```python
from build123d import *

# Parameters (mm, degrees)
SKETCH1_W                  = 38.1
SKETCH1_H                  = 127
EXTRUDE1_DEPTH             = 3.175
F_4_CLEARANCE_HOLE1_D      = 3.2639
F_4_CLEARANCE_HOLE1_DEPTH  = 101.6
F_4_CLEARANCE_HOLE1_TIP    = 0.980574487
SKETCH4_W                  = 6.35
SKETCH4_H                  = 19.05
CUT_EXTRUDE1_DEPTH         = 79.60930686
TAP_DRILL_FOR_6_TAP1_D     = 2.7051
TAP_DRILL_FOR_6_TAP1_DEPTH = 3.302
TAP_DRILL_FOR_6_TAP1_TIP   = 0.81269403
FILLET1_R                  = 6.35


with BuildPart() as part:
    # Sketch1 → Extrude1 (new body)
    with BuildSketch(Plane(origin=(0, 0, 0), x_dir=(1, 0, 0), z_dir=(0, 1, 0))):
        with Locations((0, -12.7)):
            Rectangle(SKETCH1_W, SKETCH1_H)
    extrude(amount=EXTRUDE1_DEPTH)

    # #4 Clearance Hole1
    with Locations(Plane(origin=(-10.8585, 0, 28.575), x_dir=(0, 0, -1), z_dir=(0, -1, 0))):
        with Locations((0, 0), (0, 21.717), (-38.1, 0), (-38.1, 21.717)):
            Hole(F_4_CLEARANCE_HOLE1_D / 2, depth=F_4_CLEARANCE_HOLE1_DEPTH)
            with Locations((0, 0, -(F_4_CLEARANCE_HOLE1_DEPTH + F_4_CLEARANCE_HOLE1_TIP / 2))):  # 118° drill point
                Cone(0, F_4_CLEARANCE_HOLE1_D / 2, F_4_CLEARANCE_HOLE1_TIP, mode=Mode.SUBTRACT)

    # Sketch4 → Cut-Extrude1 (cut, through all)
    with BuildSketch(Plane.XZ):
        with Locations((-15.875, -41.275)):
            Rectangle(SKETCH4_W, SKETCH4_H)
        with Locations((15.875, -41.275)):
            Rectangle(SKETCH4_W, SKETCH4_H)
    extrude(amount=-CUT_EXTRUDE1_DEPTH, mode=Mode.SUBTRACT)

    # Tap Drill for #6 Tap1
    with Locations(Plane(origin=(-6.35, 3.175, -38.1), x_dir=(0, 0, 1), z_dir=(0, 1, 0))):
        with Locations((0, 0), (0, 12.7)):
            Hole(TAP_DRILL_FOR_6_TAP1_D / 2, depth=TAP_DRILL_FOR_6_TAP1_DEPTH)
            with Locations((0, 0, -(TAP_DRILL_FOR_6_TAP1_DEPTH + TAP_DRILL_FOR_6_TAP1_TIP / 2))):  # 118° drill point
                Cone(0, TAP_DRILL_FOR_6_TAP1_D / 2, TAP_DRILL_FOR_6_TAP1_TIP, mode=Mode.SUBTRACT)

    # Fillet1
    fillet1_edges = [part.edges().sort_by_distance(p)[0] for p in [
        (-12.7, 1.5875, -31.75),
        (12.7, 1.5875, -31.75),
    ]]
    fillet(fillet1_edges, radius=FILLET1_R - 0.0001)  # a hair under: the kernel refuses the full size


solid = part.part
```
The listing builds one solid part. Answer for the finished solid, in the listing's coordinates (mm). A direction names the side the tool comes from. Give positions to 0.01 mm unless a question says otherwise; leave off trailing zeros. Order: outer loops, then holes, each group sorted by start corner. A loop starts at its lowest first (then second) coordinate and runs counter-clockwise, first axis right, second up. Notation, with made-up numbers: (-23.75, 80) -> (-14.75, 80) arc R26 cw to (-14.75, 115) -> close; hole circle Ø7 at (40, 11). An arc over 180 degrees is marked (long way). Write each question's results on one line, items separated by ' | '.
Q1. The part is cut by section A-A, the plane x = -6.35. Give the vertices of the cut face in (y, z) (3 decimals), and give its area (3 significant figures).
Checked values:
outline: (0, -50.8) -> (3.175, -50.8) -> (3.175, -39.453) -> (0, -39.453) -> close; (0, -36.747) -> (3.175, -36.747) -> (3.175, 76.2) -> (0, 76.2) -> close | area: 395 mm^2
Q2. Straight lines are drawn through the part: probe 1 along Z at (x, y) = (-9.5, 2.65); probe 2 along X at (y, z) = (1.5, -41.5); probe 3 along Z at (x, y) = (12, 2.05). For each, find the intervals that lie inside material, in ascending order. Write a range as from..to.
Checked values:
probe 1: z = -50.8..27.67, 29.48..65.77, 67.58..76.2 | probe 2: x = -12.7..12.7 | probe 3: z = -50.8..27.41, 29.74..65.51, 67.84..76.2
Q3. The part is cut by section B-B, the plane y = 1.9. State how many separate pieces and enclosed holes the cut face has, and give its area (3 significant figures).
Checked values:
separate pieces: 1 | enclosed holes: 6 | area: 4,570 mm^2
Q4. The part is cut by section C-C, the plane x = -14. Give the vertices of the cut face in (y, z) (3 decimals).
Checked values:
outline: (0, -34.25) -> (3.175, -34.25) -> (3.175, 76.2) -> (0, 76.2) -> close
Q5. Which of the six approach directions +Z, -Z, +X, -X, +Y, -Y give full straight-line access (tool end or side, diameter ignored) to faces 5 (the face through (12.7, 2, -45)), 6 (the face through (-12.7, 2, -45)), 7 (the face through (-19.05, 2, 23))?
Checked values:
face 5: -Z, +X, +Y, -Y | face 6: -Z, -X, +Y, -Y | face 7: +Z, -Z, -X, +Y, -Y
Q6. Determine the mould class of faces 1 (the face through (-6.87, 1.57, -39.35)), 2 (the face through (-14.61, 1.61, -33.56)), 3 (the face through (14.61, 1.61, -33.56)), 4 (the face through (0, 0, 12)) for opening direction X: pulls with the +X half, pulls with the -X half, needs draft (parallel to the pull), parting line crosses it, or undercut.
Checked values:
face 1: undercut | face 2: pulls with the -X half | face 3: pulls with the +X half | face 4: needs draft
Q7. Each of these flat-tipped pins is pushed along its axis until it touches: P1, Ø2, axis at x = 6.35, z = -38.1, coming from the +Y side; P2, Ø1, axis at y = 2, z = -47.5, coming from the -X side. Where does it stop, or does it pass through?
Checked values:
P1: passes through | P2: stops at x = -12.7
Q8. The part is cut by section D-D, the plane z = -34.5. Give the vertices of the cut face in (x, y) (3 decimals).
Checked values:
outline: (-13.819, 0) -> (13.819, 0) -> (13.819, 3.175) -> (-13.819, 3.175) -> close
